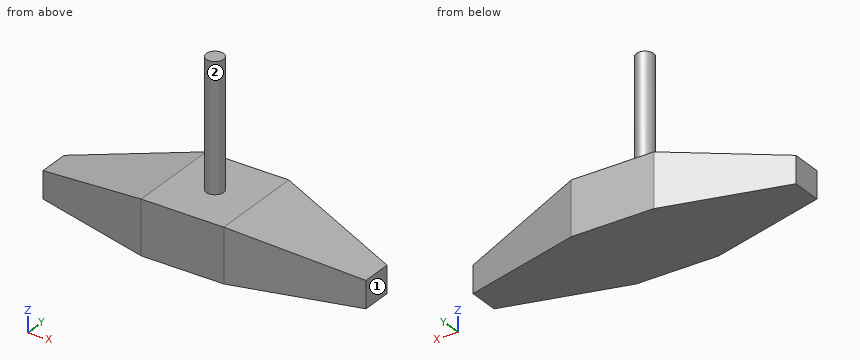
```python
from build123d import *

# Parameters (mm, degrees)
F1_DEPTH = 76.2
F2_R     = 7.014916
F3_DEPTH = 101.6
F5_DEPTH = 76.2
F6_DEPTH = 76.2


with BuildPart() as f1:
    # F0 (on Front) → F1 (new body)
    with BuildSketch(Plane.XZ):
        Polygon((129.538909, 0), (33.115212, 21.670986), (14.60965, 21.670986), (0, 21.670986), (-33.115212, 21.670986), (-129.538909, 0), (-129.538909, -21.670986), (129.538909, -21.670986), align=None)
    extrude(amount=F1_DEPTH)

    # F2 (on face) → F3 (join)
    with BuildSketch(Plane.XY.offset(21.670986)):
        with Locations((0, -38.1)):
            Circle(F2_R)
    extrude(amount=F3_DEPTH)

    # F4 (on face) → F5 (cut)
    with BuildSketch(Plane.XY.offset(21.670986)):
        Polygon((134.795412, 6.28761), (33.115212, 0), (134.795412, -27.191089), align=None)
    extrude(amount=-F5_DEPTH, mode=Mode.SUBTRACT)

    # F4 (on face) → F6 (cut)
    with BuildSketch(Plane.XY.offset(21.670986)):
        Polygon((134.795412, 6.28761), (33.115212, 0), (134.795412, -27.191089), align=None)
        Polygon((-134.795412, -27.191089), (-33.115212, 0), (-134.795412, 6.28761), align=None)
        Polygon((134.795412, -49.008911), (33.115212, -76.2), (134.795412, -82.48761), align=None)
        Polygon((-134.795412, -82.48761), (-33.115212, -76.2), (-134.795412, -49.008911), align=None)
    extrude(amount=-F6_DEPTH, mode=Mode.SUBTRACT)


solid = f1.part
```
The model under review builds one solid part; all positions refer to its coordinate system, in mm. Face numbers are marked on the shaded views. A direction names the side the tool comes from. Round coordinates to 2 decimals unless told otherwise and drop trailing zeros. Write each loop counter-clockwise with the first axis right and the second up, starting at its lowest first coordinate (ties: lowest second). Pieces come first, ordered by that corner, then holes. Notation, with made-up numbers: (-30.75, 44) - (19.25, 44) arc R24 ccw to (19.25, 71) - close; hole circle Ø10 at (76.25, 55). An arc over 180 degrees is marked (long way). Answer as CSV lines item,"result". Start each with the question number.
(1) We need section C-C on y = -38.1. State the section outline as (x, z) points.
(2) For the marked faces 1 and 2, list the 3-axis set-ups (+Z, -Z, +X, -X, +Y, -Y) from which the entire face can be reached by the end or side of a thin tool; tool diameter is ignored.
(3) We need section D-D on z = 86.5. State the section outline as (x, y) points.
(4) We need section B-B on x = 0. State the section outline as (y, z) points, plus the area to 3 significant figures.
(5) We need section A-A on z = -12.5. State the section outline as (x, y) points.
(6) For pin 1 Ø10 at (y, z) = (-36.5, 91.5) entering from +X; pin 2 Ø1 at (x, y) = (32, -9) entering from +Z, all flat-tipped, find the tip position at first contact; note any pin that passes through.
(7) To check wall thickness, follow line 1 (Z direction, x = -1, y = -3.5); line 2 (Z direction, x = 42, y = -52.5); line 3 (X direction, y = -32, z = 86). State the ranges of each line that lie inside material, in increasing order.
Worked answers:
1,outline,"(-129.54, -21.67) - (129.54, -21.67) - (129.54, 0) - (33.12, 21.67) - (7.01, 21.67) - (7.01, 123.27) - (-7.01, 123.27) - (-7.01, 21.67) - (-33.12, 21.67) - (-129.54, 0) - close"
2,face 1,"+Z, -Z, +X, +Y, -Y"
2,face 2,"+Z"
3,outline,"circle Ø14.03 at (0, -38.1)"
4,outline,"(-76.2, -21.67) - (0, -21.67) - (0, 21.67) - (-31.09, 21.67) - (-31.09, 123.27) - (-45.11, 123.27) - (-45.11, 21.67) - (-76.2, 21.67) - close"
4,area,"4,730 mm²"
5,outline,"(-129.54, -50.41) - (-33.12, -76.2) - (33.12, -76.2) - (129.54, -50.41) - (129.54, -25.79) - (33.12, 0) - (-33.12, 0) - (-129.54, -25.79) - close"
6,pin 1,"x = 7.01"
6,pin 2,"z = 21.67"
7,line 1,"-21.67 to 21.67"
7,line 2,"-21.67 to 19.67"
7,line 3,"-3.46 to 3.46"
